Geometry check sheet. Reference: drawing and pictorial views, mm from the part's lowest x, y, z. Round coordinates to 2 decimals unless told otherwise and drop trailing zeros. Write each loop counter-clockwise with the first axis right and the second up, starting at its lowest first coordinate (ties: lowest second). Pieces come first, ordered by that corner, then holes. Notation, with made-up numbers: M -34,37 L 19,37 A29 cw 19,61 Z; hole C 61,81 d10. An arc over 180 degrees is marked long. Put each result on its own line as item: value. Start each with the question number.
(1) Section check A-A on x = 134. Record the cut outline in (y, z), then the cut area to 3 significant figures.
(2) Gauge pin test, flat end, axial feed: pin 1 (12.5 mm diameter, centred on x = 62, z = 26, fed in from +Y). Record the tip position at first contact, or that the pin passes through.
(3) Section check C-C on y = 3.6. Record the cut outline in (x, z) (3 decimals).
(4) Mould release check, pull along X, two halves, no side actions. Record for the marked faces 1 and 2: pulls with the +X half, pulls with the -X half, needs draft (parallel to the pull), parting line crosses it, or undercut.
(5) Material ranges on probe 1 along Z at (x, y) = (38, 3.2); probe 2 along X at (y, z) = (1.4, 8) (3 decimals); probe 3 along X at (y, z) = (4.4, 31.5) (3 decimals), recorded low to high.
(6) Section check B-B on z = 27. Record the cut outline in (x, y) (3 decimals).
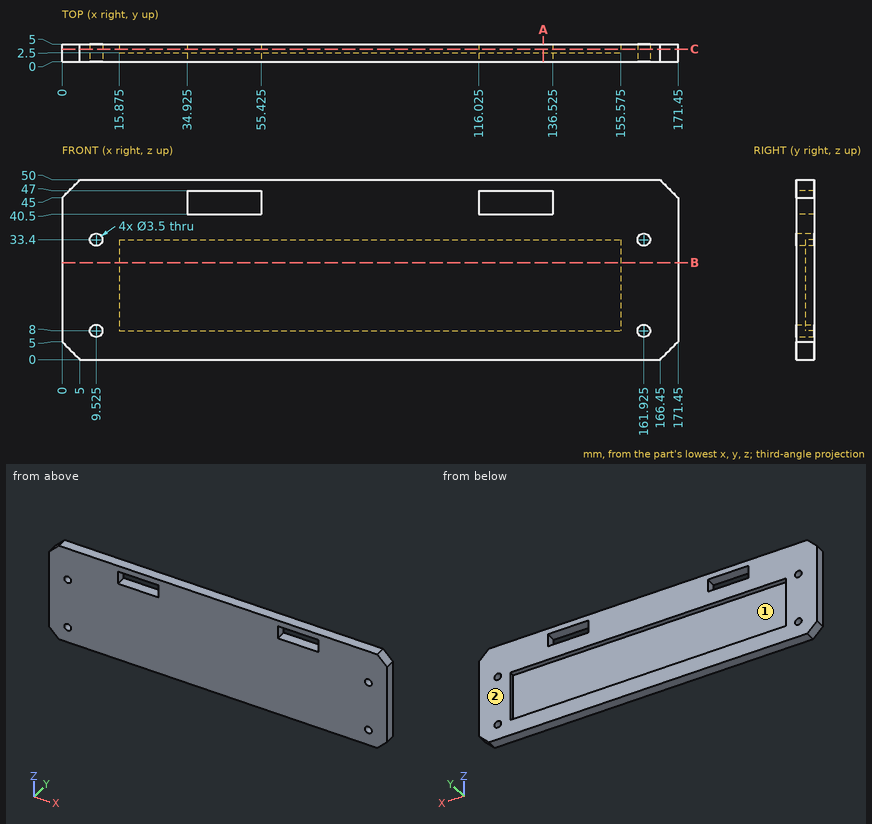
Answers follow:
1. outline: M 0,0 L 5,0 L 5,8 L 2.5,8 L 2.5,33.4 L 5,33.4 L 5,40.5 L 0,40.5 Z; M 0,47 L 5,47 L 5,50 L 0,50 Z
1. area: 154 mm^2
2. pin 1: stops at y = 2.5
3. outline: M 0,5 L 5,0 L 166.45,0 L 171.45,5 L 171.45,45 L 166.45,50 L 5,50 L 0,45 Z; hole C 9.525,8 d3.5; hole C 9.525,33.4 d3.5; hole M 15.875,8 L 155.575,8 L 155.575,33.4 L 15.875,33.4 Z; hole M 34.925,40.5 L 55.425,40.5 L 55.425,47 L 34.925,47 Z; hole M 116.025,40.5 L 136.525,40.5 L 136.525,47 L 116.025,47 Z; hole C 161.925,8 d3.5; hole C 161.925,33.4 d3.5
4. face 1: undercut
4. face 2: needs draft
5. probe 1: z = 0 to 8, 33.4 to 40.5, 47 to 50
5. probe 2: x = 0 to 7.775, 11.275 to 160.175, 163.675 to 171.45
5. probe 3: x = 0 to 15.875, 155.575 to 171.45
6. outline: M 0,0 L 171.45,0 L 171.45,5 L 155.575,5 L 155.575,2.5 L 15.875,2.5 L 15.875,5 L 0,5 Z
